Can you work these out from the model? Positions are in its coordinate system, mm. Face numbers are marked on the shaded views. A direction names the side the tool comes from. Round coordinates to 2 decimals unless told otherwise and drop trailing zeros. Write each loop counter-clockwise with the first axis right and the second up, starting at its lowest first coordinate (ties: lowest second). Pieces come first, ordered by that corner, then holes. Notation, with made-up numbers: (84.5, 43.5) -> (114.5, 43.5) arc R31 ccw to (114.5, 77.5) -> close; hole circle Ø1 at (87.25, 1). An arc over 180 degrees is marked (long way). Write item = value, one per line. Start each with the question number.
1) Imagine slicing it at C-C, the plane y = -119. Please give me the cut outline in (x, z).
2) For the marked faces 1 and 2, which set-ups out of +Z, -Z, +X, -X, +Y, -Y let a thin tool reach every point of the face, with its end or its side?
3) If I drill on line 1 (Y direction, x = 13.5, z = 6.5); line 2 (Y direction, x = 5, z = 0.5); line 3 (Z direction, x = 0, y = -149), over which ranges is the centre line in solid material (lowest first)?
4) Imagine slicing it at A-A, the plane x = 9. Please give me the cut outline in (y, z).
5) Imagine slicing it at B-B, the plane z = 11. Please give me the cut outline in (x, y).
6) I'm going to push flat-ended pins straight in: pin 1 (3 mm diameter, centred on y = -138, z = 1.5, fed in from -X); pin 2 (3 mm diameter, centred on x = -10, y = -78, fed in from +Z); pin 3 (3.5 mm diameter, centred on x = 0.59, z = -0.56, fed in from -Y). Where does each tip first touch, or does it pass through?
7) Imagine slicing it at D-D, the plane z = 0. Please give me the cut outline in (x, y) (3 decimals), then the cut area to 3 significant figures.
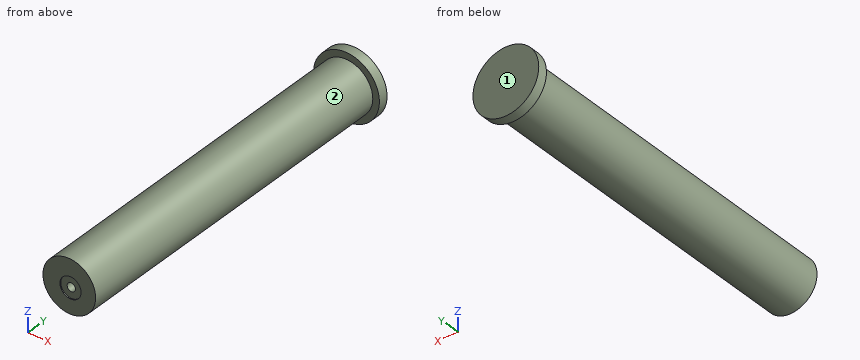
Autodesk Inventor part; units mm, degrees
ref_plane "YZ Plane" through (0, 0, 0) normal (1, 0, 0) x (0, 1, 0)
ref_plane "XZ Plane" through (0, 0, 0) normal (0, 1, 0) x (-1, 0, 0)
ref_plane "XY Plane" through (0, 0, 0) normal (0, 0, 1) x (1, 0, 0)
sketch "Boceto1" plane through (0, 0, 0) normal (0, 1, 0) x (-1, 0, 0)
  circle A0 centre (0, 0) radius 12.7
  circle A1 centre (0, 0) radius 15.875
  dimension "d0" = 25.4
  dimension "d1" = 31.75
extrude "Extrusión1" add sketch "Boceto1" along normal blind 4.7
sketch "Boceto2" plane through (0, 4.7, 0) normal (0, 1, 0) x (1, 0, 0)
  circle A0 centre (0, 0) radius 12.7
  dimension "d4" = 25.4
extrude "Extrusión2" add sketch "Boceto2" against normal blind 173.6
hole "Agujero1" at (0.5939, -168.9, -0.5568) direction (0, 1, 0) diameter 4 depth 8 counterbore diameter 10.2 counterbore depth 0.5
thread "Rosca1"
properties part number "post"
Reported:
q1.outline = circle Ø25.4 at (0, 0)
q2.face_1 = +Z, -Z, +X, -X, +Y
q2.face_2 = -Y
q3.line_1 = 0 to 4.7
q3.line_2 = -168.4 to 4.7
q3.line_3 = -12.7 to 12.7
q4.outline = (-168.9, -8.96) -> (0, -8.96) -> (0, -13.08) -> (4.7, -13.08) -> (4.7, 13.08) -> (0, 13.08) -> (0, 8.96) -> (-168.9, 8.96) -> close
q5.outline = (-11.45, 0) -> (-6.35, 0) -> (-6.35, -168.9) -> (6.35, -168.9) -> (6.35, 0) -> (11.45, 0) -> (11.45, 4.7) -> (-11.45, 4.7) -> close
q6.pin_1 = -12.7
q6.pin_2 = 9.44
q6.pin_3 = -160.9
q7.outline = (-15.875, 0) -> (-12.7, 0) -> (-12.7, -168.9) -> (-4.476, -168.9) -> (-4.476, -168.4) -> (-1.327, -168.4) -> (-1.327, -160.9) -> (2.515, -160.9) -> (2.515, -168.4) -> (5.663, -168.4) -> (5.663, -168.9) -> (12.7, -168.9) -> (12.7, 0) -> (15.875, 0) -> (15.875, 4.7) -> (-15.875, 4.7) -> close
q7.area = 4,410 mm²
